Read the model definition and answer for the solid it produces. Units are mm, in the model's axes. A direction names the side the tool comes from. Give positions to 0.01 mm unless a question says otherwise; leave off trailing zeros. Order: outer loops, then holes, each group sorted by start corner. A loop starts at its lowest first (then second) coordinate and runs counter-clockwise, first axis right, second up.
```python
from build123d import *

# Parameters (mm, degrees)
ESQUISSE1_R             = 2.15
ESQUISSE1_W             = 6
ESQUISSE1_H             = 12
BOSS_EXTRU_1_DEPTH      = 9
ESQUISSE2_R             = 8
ENL_V_MAT_EXTRU_1_DEPTH = 5
ESQUISSE3_R             = 1.6
ENL_V_MAT_EXTRU_2_DEPTH = 33.878564446


with BuildPart() as part:
    # Esquisse1 → Boss.-Extru.1 (new body)
    with BuildSketch(Plane.XY):
        with BuildLine():
            Line((0, -10), (-28.284271247, -10))
            ThreePointArc((-28.284271247, -10), (-30, 0), (-28.284271247, 10))
            Line((-28.284271247, 10), (0, 10))
            Line((0, 10), (28.284271247, 10))
            ThreePointArc((28.284271247, 10), (30, 0), (28.284271247, -10))
            Line((28.284271247, -10), (0, -10))
        make_face()
        with Locations((-25, 0)):
            Circle(ESQUISSE1_R, mode=Mode.SUBTRACT)
        with Locations((25, 0)):
            Circle(ESQUISSE1_R, mode=Mode.SUBTRACT)
        with Locations((-15, 0)):
            Rectangle(ESQUISSE1_W, ESQUISSE1_H, mode=Mode.SUBTRACT)
        with Locations((15, 0)):
            Rectangle(ESQUISSE1_W, ESQUISSE1_H, mode=Mode.SUBTRACT)
    extrude(amount=BOSS_EXTRU_1_DEPTH)

    # Esquisse2 → Enlèv. mat.-Extru.1 (cut)
    with BuildSketch(Plane(origin=(0, 0, 0), x_dir=(-1, 0, 0), z_dir=(0, 0, -1))):
        Circle(ESQUISSE2_R)
    extrude(amount=-ENL_V_MAT_EXTRU_1_DEPTH, mode=Mode.SUBTRACT)

    # Esquisse3 → Enlèv. mat.-Extru.2 (cut, through all)
    with BuildSketch(Plane.XY.offset(9)):
        Circle(ESQUISSE3_R)
    extrude(amount=-ENL_V_MAT_EXTRU_2_DEPTH, mode=Mode.SUBTRACT)


solid = part.part
```
1) The part is cut by section C-C on z = 7.25. Determine the outline of the cut face in (x, y).
Final values:
outline: (-28.28, -10) - (28.28, -10) arc R30 ccw to (28.28, 10) - (-28.28, 10) arc R30 ccw to start; hole circle Ø4.3 at (-25, 0); hole (-18, -6) - (-12, -6) - (-12, 6) - (-18, 6) - close; hole circle Ø3.2 at (0, 0); hole (12, -6) - (18, -6) - (18, 6) - (12, 6) - close; hole circle Ø4.3 at (25, 0)
2) Given pin 1 (4.5 mm diameter, centred on y = -2, z = 5.5, fed in from -X); pin 2 (4 mm diameter, centred on x = 25, y = 0, fed in from -Z); pin 3 (1.5 mm diameter, centred on y = -6.5, z = 7, fed in from -X); pin 4 (2 mm diameter, centred on x = -5.5, y = 2, fed in from -Z), each flat-ended and moving along its own axis, determine where each tip first touches the part or whether it passes through.
Final values:
pin 1: stops at x = -30
pin 2: passes through
pin 3: stops at x = -29.44
pin 4: stops at z = 5
3) A tool of negligible diameter and unlimited length cuts with its end or side. For faces 1 (the face through (1.73, -7.81, 2.46)), 2 (the face through (7, 5, 0)), 3 (the face through (-15, -6, 4)), from which of +Z, -Z, +X, -X, +Y, -Y can it reach the whole face along a straight path? Write none if from no direction.
Final values:
face 1: -Z
face 2: -Z, +X, -X, +Y, -Y
face 3: +Z, -Z
4) The part is cut by section D-D on y = -3.5. Determine the outline of the cut face in (x, z).
Final values:
outline: (-29.8, 0) - (-18, 0) - (-18, 9) - (-29.8, 9) - close; (-12, 0) - (-7.19, 0) - (-7.19, 5) - (7.19, 5) - (7.19, 0) - (12, 0) - (12, 9) - (-12, 9) - close; (18, 0) - (29.8, 0) - (29.8, 9) - (18, 9) - close
5) Consider L1, parallel to X at y = -4.25, z = 8.5; L2, parallel to Y at x = 0, z = 3.45; L3, parallel to Y at x = -25, z = 5.5. Determine where each line is inside the solid, lowest interval first.
Final values:
L1: x = -29.7 to -18, -12 to 12, 18 to 29.7
L2: y = -10 to -8, 8 to 10
L3: y = -10 to -2.15, 2.15 to 10
6) The part is cut by section B-B on y = 0. Determine the outline of the cut face in (x, z).
Final values:
outline: (-30, 0) - (-27.15, 0) - (-27.15, 9) - (-30, 9) - close; (-22.85, 0) - (-18, 0) - (-18, 9) - (-22.85, 9) - close; (-12, 0) - (-8, 0) - (-8, 5) - (-1.6, 5) - (-1.6, 9) - (-12, 9) - close; (1.6, 5) - (8, 5) - (8, 0) - (12, 0) - (12, 9) - (1.6, 9) - close; (18, 0) - (22.85, 0) - (22.85, 9) - (18, 9) - close; (27.15, 0) - (30, 0) - (30, 9) - (27.15, 9) - close
7) For a pull along Y with two mould halves and no side action, classify faces 4 (the face through (0, 2, 9)), 5 (the face through (0, 10, 4)), 6 (the face through (-1.27, -0.97, 7.03)), 7 (the face through (-22.95, 0.65, 4.44)) as released by +Y, released by -Y, zero draft, split by the parting line, or undercut.
Final values:
face 4: zero draft
face 5: released by +Y
face 6: undercut
face 7: undercut
8) The part is cut by section A-A on x = 0. Determine the outline of the cut face in (y, z), and give its area (3 significant figures).
Final values:
outline: (-10, 0) - (-8, 0) - (-8, 5) - (-1.6, 5) - (-1.6, 9) - (-10, 9) - close; (1.6, 5) - (8, 5) - (8, 0) - (10, 0) - (10, 9) - (1.6, 9) - close
area: 87.2 mm2
